CAD build for the part. Positions are in the model's coordinates, mm. A direction names the side the tool comes from. Round coordinates to 2 decimals unless told otherwise and drop trailing zeros. Write each loop counter-clockwise with the first axis right and the second up, starting at its lowest first coordinate (ties: lowest second). Pieces come first, ordered by that corner, then holes. Notation, with made-up numbers: (87.25, -4) - (145.25, -4) arc R32 cw to (145.25, 31) - close; hole circle Ø9 at (44.5, -24.75). An arc over 180 degrees is marked (long way). Answer in a Markdown table with one row per item.
```python
from build123d import *

# Parameters (mm, degrees)
F0_R     = 4.55
F1_DEPTH = 12
F2_SIZE2 = 0.5
F2_SIZE  = 5
F3_R     = 6.5
F3_R_2   = 4.55
F4_DEPTH = 4
F5_R     = 1


with BuildPart() as f1:
    # F0 (on Top) → F1 (new body)
    with BuildSketch(Plane.XY):
        Circle(F0_R)
    extrude(amount=F1_DEPTH)

    # F2
    f2_edges = [f1.edges().sort_by_distance(p)[0] for p in [
        (-4.55, 0, 0),
    ]]
    chamfer(f2_edges, length=F2_SIZE, length2=F2_SIZE2)

    # F3 (on face) → F4 (join)
    with BuildSketch(Plane.XY.offset(12)):
        Circle(F3_R)
        Circle(F3_R_2, mode=Mode.SUBTRACT)
        Circle(F3_R_2)
    extrude(amount=F4_DEPTH)

    # F5
    f5_edges = [f1.edges().sort_by_distance(p)[0] for p in [
        (-6.5, 0, 16),
    ]]
    fillet(f5_edges, radius=F5_R)


solid = f1.part
```
Q1. Saw through at A-A on y = 0. List the corners of the cut face in (x, z).
Computed:
| item | result |
|---|---|
| outline | (-6.5, 12) - (-4.55, 12) - (-4.55, 5) - (-4.05, 0) - (4.05, 0) - (4.55, 5) - (4.55, 12) - (6.5, 12) - (6.5, 15) arc R1 ccw to (5.5, 16) - (-5.5, 16) arc R1 ccw to (-6.5, 15) - close |
Q2. 3-axis set-ups, long thin cutter, end or side, ignore diameter. For faces 1 (the cylindrical face through (-0.99, -4.44, 8.45)), 2 (the flat face through (0, 0, 0)): which of +Z, -Z, +X, -X, +Y, -Y reach the whole face in a straight line?
Computed:
| item | result |
|---|---|
| face 1 | -Z |
| face 2 | -Z, +X, -X, +Y, -Y |
Q3. Drill centre lines: line 1 (Z direction, x = 5, y = -1.75); line 2 (X direction, y = -1.25, z = 15.25); line 3 (Y direction, x = -1.5, z = 13.75). Where is each one in solid material? Low to high.
Computed:
| item | result |
|---|---|
| line 1 | z = 12 to 16 |
| line 2 | x = -6.35 to 6.35 |
| line 3 | y = -6.32 to 6.32 |
Q4. Flat gauge pins, fed straight in: pin 1 (2 mm diameter, centred on x = -3.5, z = 7, fed in from +Y); pin 2 (1 mm diameter, centred on y = 3.5, z = 12.5, fed in from -X); pin 3 (3 mm diameter, centred on x = 2, z = 11.5, fed in from +Y); pin 4 (4 mm diameter, centred on x = 2, y = 1, fed in from -Z). Where does each tip first touch, or does it go through?
Computed:
| item | result |
|---|---|
| pin 1 | stops at y = 3.8 |
| pin 2 | stops at x = -5.77 |
| pin 3 | stops at y = 6.47 |
| pin 4 | stops at z = 0 |
Q5. Saw through at C-C on z = 1.5. List the corners of the cut face in (x, y).
Computed:
| item | result |
|---|---|
| outline | circle Ø8.4 at (0, 0) |
